Build history of the part. All positions in model axes, mm. Face numbers are marked on the shaded views. A direction names the side the tool comes from. Round coordinates to 2 decimals unless told otherwise and drop trailing zeros. Write each loop counter-clockwise with the first axis right and the second up, starting at its lowest first coordinate (ties: lowest second). Pieces come first, ordered by that corner, then holes. Notation, with made-up numbers: (-7.5, 64) -> (9.5, 64) arc R4 cw to (9.5, 71) -> close; hole circle Ø9 at (7.25, -5.75). An arc over 180 degrees is marked (long way). Return JSON: item names as keys, results as strings.
from build123d import *

# Parameters (mm, degrees)
EXTRUDE_THIN1_DEPTH      = 40.64
BOSS_EXTRUDE2_DEPTH      = 2.54
BOSS_EXTRUDE2_DEPTH_BACK = 5.08
SKETCH7_W                = 25.274399357
SKETCH7_H                = 76.2
SKETCH10_W               = 25.274399357
SKETCH10_H               = 1.587143393
CUT_EXTRUDE10_DEPTH      = 31.75


with BuildPart() as part:
    # Sketch1 → Extrude-Thin1 (new body)
    with BuildSketch(Plane(origin=(0, 0, 0), x_dir=(1, 0, 0), z_dir=(0, 1, 0))):
        Polygon((-25.4, 25.4), (0, 25.4), (0, 0), (-25.4, 0), (-25.4, -2.54), (2.54, -2.54), (2.54, 27.94), (-25.4, 27.94), align=None)
    extrude(amount=EXTRUDE_THIN1_DEPTH)

    # Sketch7 → Boss-Extrude2 (add, two sides: drawn at the far end of the back side and taken through both)
    with BuildSketch(Plane.XY.offset(2.54).offset(-BOSS_EXTRUDE2_DEPTH_BACK)):
        with Locations((15.177199679, 2.54)):
            Rectangle(SKETCH7_W, SKETCH7_H)
    extrude(amount=BOSS_EXTRUDE2_DEPTH + BOSS_EXTRUDE2_DEPTH_BACK)

    # Sketch10 → Cut-Extrude10 (cut)
    with BuildSketch(Plane.XZ.offset(35.56)):
        with Locations((15.177199679, 1.746428304)):
            Rectangle(SKETCH10_W, SKETCH10_H)
    extrude(amount=-CUT_EXTRUDE10_DEPTH, mode=Mode.SUBTRACT)


solid = part.part
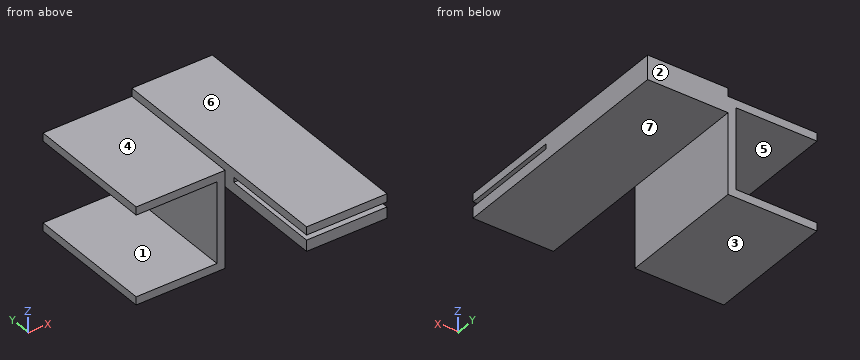
Q1. Saw through at C-C on z = -1. List the corners of the cut face in (x, y), then the cut area to 3 significant figures.
Verdict:
{"outline": "(0, 0) -> (2.54, 0) -> (2.54, -35.56) -> (27.81, -35.56) -> (27.81, 40.64) -> (0, 40.64) -> close", "area": "2,030 mm²"}
Q2. Saw through at A-A on x = -2. List the corners of the cut face in (y, z).
Verdict:
{"outline": "(0, -27.94) -> (40.64, -27.94) -> (40.64, -25.4) -> (0, -25.4) -> close; (0, 0) -> (40.64, 0) -> (40.64, 2.54) -> (0, 2.54) -> close"}
Q3. 3-axis set-ups, long thin cutter, end or side, ignore diameter. For the marked faces 4, 5, 6 and 7: which of +Z, -Z, +X, -X, +Y, -Y reach the whole face in a straight line?
Verdict:
{"face 4": "+Z, -X, +Y, -Y", "face 5": "-X, +Y, -Y", "face 6": "+Z, +X, -X, +Y, -Y", "face 7": "-Z, +X, +Y, -Y"}
Q4. Wall check: L1, parallel to Z at x = -8.5, y = 22; L2, parallel to X at y = 29, z = -1; L3, parallel to Z at x = 18.5, y = 0.5. Give the ranges that are in metal, low to high.
Verdict:
{"L1": "z = -27.94 to -25.4, 0 to 2.54", "L2": "x = 0 to 27.81", "L3": "z = -2.54 to 5.08"}
Q5. Saw through at D-D on y = 30.5. List the corners of the cut face in (x, z), then the cut area to 3 significant figures.
Verdict:
{"outline": "(-25.4, -27.94) -> (2.54, -27.94) -> (2.54, -2.54) -> (27.81, -2.54) -> (27.81, 5.08) -> (2.54, 5.08) -> (2.54, 2.54) -> (-25.4, 2.54) -> (-25.4, 0) -> (0, 0) -> (0, -25.4) -> (-25.4, -25.4) -> close", "area": "399 mm²"}
Q6. Pin check, flat tips, straight feed: pin 1 Ø8.5 at (x, z) = (-4.5, -11.5) entering from -Y; pin 2 Ø12.5 at (y, z) = (25, -16.5) entering from +X; pin 3 Ø7.5 at (y, z) = (23, -9.5) entering from -X; pin 4 Ø7.5 at (x, y) = (-7, 20.5) entering from +Z. Stop position of each tip, or through.
Verdict:
{"pin 1": "passes through", "pin 2": "stops at x = 2.54", "pin 3": "stops at x = 0", "pin 4": "stops at z = 2.54"}
Q7. Two-plate mould, pull along Z, no slides. Class the marked faces 1, 2 and 3: +Z half, -Z half, draft (parallel to the pull), parting line (faces both ways), or undercut.
Verdict:
{"face 1": "undercut", "face 2": "draft", "face 3": "-Z half"}
Q8. Saw through at B-B on y = -10.5. List the corners of the cut face in (x, z).
Verdict:
{"outline": "(2.54, -2.54) -> (27.81, -2.54) -> (27.81, 0.95) -> (2.54, 0.95) -> close; (2.54, 2.54) -> (27.81, 2.54) -> (27.81, 5.08) -> (2.54, 5.08) -> close"}
